Input: part model. Units: mm. Frame: model coordinates. A direction names the side the tool comes from. Coordinates: 2 decimals unless noted, no trailing zeros. Loops run counter-clockwise (first coordinate to the right, second up) from the corner with the lowest first, then second, coordinate; pieces in that order, holes last. Notation, with made-up numbers: M 0.25,43.5 L 37.25,43.5 A23 cw 37.25,75.5 Z; hole C -13.5,39 d3. An arc over 180 degrees is marked long. Use a Markdown table: item, result. Add a question column.
1. Set-up query: faces 1 (the flat face through (-42, -38.1, 0)), 2 (the flat face through (20, -40, 0)), 3 (the flat face through (-63.5, -29, 0)), 4 (the flat face through (-62, 20.127, 0)), 5 (the flat face through (62, -20.127, 0)). Return all of +Z, -Z, +X, -X, +Y, -Y with unobstructed straight access to the full face (end or side cutting, diameter ignored); none if empty.
2. Line query: L1, parallel to Y at x = -45, z = -0.2; L2, parallel to X at y = 3, z = -0.8. Output: solid intervals per line, ascending. Write a range as [from, to].
3. Section B-B on y = -7. Output: boundary loops of the cut face in (x, z), then the cut area to 3 significant figures.
4. Section C-C on x = -47. Output: boundary loops of the cut face in (y, z).
5. Draft query along Y for faces 6 (the flat face through (63.5, -29, 0)), 7 (the flat face through (-60.452, 0, 0)), 8 (the flat face through (41, -38.1, 0)). Return one class per face: +Y half, -Y half, draft (parallel to the pull), parting line (faces both ways), or undercut.
6. Section A-A on z = 0.8. Output: boundary loops of the cut face in (x, y).
7. Pin query (flat end, axial travel): pin 1 (1 mm diameter, centred on y = 16.5, z = 0, fed in from +X); pin 2 (0.9 mm diameter, centred on y = -39.5, z = 0, fed in from +X); pin 3 (1.5 mm diameter, centred on y = -40, z = -0.5, fed in from -X). Return the tip coordinate at first contact, or that it passes through.
```python
from build123d import *

# Parameters (mm, degrees)
SKETCH1_W           = 127
SKETCH1_H           = 76.2
BOSS_EXTRUDE1_DEPTH = 1.4986
SKETCH2_W           = 3.048
SKETCH2_H           = 40.254
SKETCH2_W_2         = 40.254
SKETCH2_H_2         = 2.9464
CUT_EXTRUDE1_DEPTH  = 3.9972
SKETCH3_W           = 40
SKETCH3_H           = 2.9464
BOSS_EXTRUDE2_DEPTH = 2.9972


with BuildPart() as part:
    # Sketch1 → Boss-Extrude1 (new body, symmetric)
    with BuildSketch(Plane.XY):
        Rectangle(SKETCH1_W, SKETCH1_H)
    extrude(amount=BOSS_EXTRUDE1_DEPTH, both=True)

    # Sketch2 → Cut-Extrude1 (cut, through all)
    with BuildSketch(Plane.XY.offset(1.4986)):
        with Locations((-61.976, 0)):
            Rectangle(SKETCH2_W, SKETCH2_H)
        with Locations((61.976, 0)):
            Rectangle(SKETCH2_W, SKETCH2_H)
        with Locations((0, -39.5732)):
            Rectangle(SKETCH2_W_2, SKETCH2_H_2)
    extrude(amount=-CUT_EXTRUDE1_DEPTH, mode=Mode.SUBTRACT)

    # Sketch3 → Boss-Extrude2 (add, through all)
    with BuildSketch(Plane.XY.offset(1.4986)):
        with Locations((0, -39.5732)):
            Rectangle(SKETCH3_W, SKETCH3_H)
    extrude(amount=-BOSS_EXTRUDE2_DEPTH)


solid = part.part
```
Answers below:
| question | item | result |
|---|---|---|
| 1 | face 1 | +Z, -Z, -X, -Y |
| 1 | face 2 | +Z, -Z, +X, -Y |
| 1 | face 3 | +Z, -Z, -X, +Y, -Y |
| 1 | face 4 | +Z, -Z, -X |
| 1 | face 5 | +Z, -Z, +X |
| 2 | L1 | y = [-38.1, 38.1] |
| 2 | L2 | x = [-60.45, 60.45] |
| 3 | outline | M -60.45,-1.5 L 60.45,-1.5 L 60.45,1.5 L -60.45,1.5 Z |
| 3 | area | 362 mm² |
| 4 | outline | M -38.1,-1.5 L 38.1,-1.5 L 38.1,1.5 L -38.1,1.5 Z |
| 5 | face 6 | draft |
| 5 | face 7 | undercut |
| 5 | face 8 | -Y half |
| 6 | outline | M -63.5,-38.1 L -20,-38.1 L -20,-41.05 L 20,-41.05 L 20,-38.1 L 63.5,-38.1 L 63.5,-20.13 L 60.45,-20.13 L 60.45,20.13 L 63.5,20.13 L 63.5,38.1 L -63.5,38.1 L -63.5,20.13 L -60.45,20.13 L -60.45,-20.13 L -63.5,-20.13 Z |
| 7 | pin 1 | stops at x = 60.45 |
| 7 | pin 2 | stops at x = 20 |
| 7 | pin 3 | stops at x = -20 |
